Work out the finished part from the listing and answer in its coordinate system (mm). Coordinates: 2 decimals unless noted, no trailing zeros. Answer as a JSON object with one key per item and string values. Group by question number.
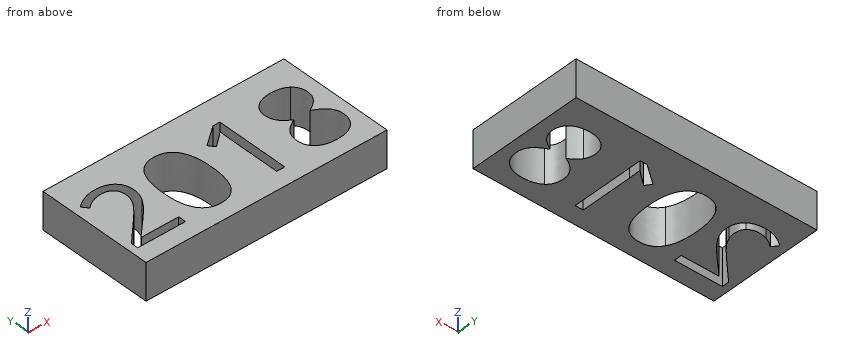
from build123d import *

# Parameters (mm, degrees)
F0_W     = 131.467973601
F0_H     = 63
F1_DEPTH = 20


with BuildPart() as f1:
    # F0 (on Top) → F1 (new body)
    with BuildSketch(Plane.XY):
        with Locations((-65.7339868005, -31.5)):
            Rectangle(F0_W, F0_H)
        with BuildLine():
            Line((-101.4531498872, -49.3273232344), (-101.4531498872, -53.5062699422))
            Line((-101.4531498872, -53.5062699422), (-127.5433306843, -53.5062699422))
            Line((-127.5433306843, -53.5062699422), (-127.5433306843, -49.6227165568))
            Line((-127.5433306843, -49.6227165568), (-117.0916198954, -39.1188775346))
            add(Edge.make_bspline(
                [(-117.0916198954, -39.1188775346), (-112.313198504, -34.279639871), (-110.7927916977, -32.2162306338)],
                knots=[0, 0, 0, 1, 1, 1], degree=2))
            add(Edge.make_bspline(
                [(-110.7927916977, -32.2162306338), (-109.2723848913, -30.1528213966), (-108.5121814882, -28.1980126456)],
                knots=[0, 0, 0, 1, 1, 1], degree=2))
            add(Edge.make_bspline(
                [(-108.5121814882, -28.1980126456), (-107.751978085, -26.2432038945), (-107.751978085, -23.9930018211)],
                knots=[0, 0, 0, 1, 1, 1], degree=2))
            add(Edge.make_bspline(
                [(-107.751978085, -23.9930018211), (-107.751978085, -20.8131795861), (-109.6807227193, -18.9539392629)],
                knots=[0, 0, 0, 1, 1, 1], degree=2))
            add(Edge.make_bspline(
                [(-109.6807227193, -18.9539392629), (-111.6094673537, -17.0946989397), (-115.0325546777, -17.0946989397)],
                knots=[0, 0, 0, 1, 1, 1], degree=2))
            add(Edge.make_bspline(
                [(-115.0325546777, -17.0946989397), (-117.4999577234, -17.0946989397), (-119.7154076413, -17.9113745957)],
                knots=[0, 0, 0, 1, 1, 1], degree=2))
            add(Edge.make_bspline(
                [(-119.7154076413, -17.9113745957), (-121.9308575591, -18.7280502517), (-124.6415256938, -20.8739958584)],
                knots=[0, 0, 0, 1, 1, 1], degree=2))
            Line((-124.6415256938, -20.8739958584), (-127.0307363895, -17.807118129))
            add(Edge.make_bspline(
                [(-127.0307363895, -17.807118129), (-121.5485838478, -13.2458977099), (-115.084682911, -13.2458977099)],
                knots=[0, 0, 0, 1, 1, 1], degree=2))
            add(Edge.make_bspline(
                [(-115.084682911, -13.2458977099), (-109.4895858637, -13.2458977099), (-106.3141076481, -16.1086065253)],
                knots=[0, 0, 0, 1, 1, 1], degree=2))
            add(Edge.make_bspline(
                [(-106.3141076481, -16.1086065253), (-103.1386294325, -18.9713153407), (-103.1386294325, -23.8018649655)],
                knots=[0, 0, 0, 1, 1, 1], degree=2))
            add(Edge.make_bspline(
                [(-103.1386294325, -23.8018649655), (-103.1386294325, -27.5811618841), (-105.2585109226, -31.2735784139)],
                knots=[0, 0, 0, 1, 1, 1], degree=2))
            add(Edge.make_bspline(
                [(-105.2585109226, -31.2735784139), (-107.3783924126, -34.9659949436), (-113.1820023934, -40.6132202243)],
                knots=[0, 0, 0, 1, 1, 1], degree=2))
            Line((-113.1820023934, -40.6132202243), (-121.8700412868, -49.1101222621))
            Line((-121.8700412868, -49.1101222621), (-121.8700412868, -49.3273232344))
            Line((-121.8700412868, -49.3273232344), (-101.4531498872, -49.3273232344))
        make_face(mode=Mode.SUBTRACT)
        with BuildLine():
            add(Edge.make_bspline(
                [(-72.7999976166, -18.4283129099), (-69.4464146037, -23.6715443821), (-69.4464146037, -33.6019728373)],
                knots=[0, 0, 0, 1, 1, 1], degree=2))
            add(Edge.make_bspline(
                [(-69.4464146037, -33.6019728373), (-69.4464146037, -43.897298926), (-72.6913971304, -48.9754576593)],
                knots=[0, 0, 0, 1, 1, 1], degree=2))
            add(Edge.make_bspline(
                [(-72.6913971304, -48.9754576593), (-75.9363796571, -54.0536163925), (-82.6174815662, -54.0536163925)],
                knots=[0, 0, 0, 1, 1, 1], degree=2))
            add(Edge.make_bspline(
                [(-82.6174815662, -54.0536163925), (-89.0205662307, -54.0536163925), (-92.3611171852, -48.8538251148)],
                knots=[0, 0, 0, 1, 1, 1], degree=2))
            add(Edge.make_bspline(
                [(-92.3611171852, -48.8538251148), (-95.7016681398, -43.654033837), (-95.7016681398, -33.6019728373)],
                knots=[0, 0, 0, 1, 1, 1], degree=2))
            add(Edge.make_bspline(
                [(-95.7016681398, -33.6019728373), (-95.7016681398, -23.2371424374), (-92.4697176714, -18.2111119375)],
                knots=[0, 0, 0, 1, 1, 1], degree=2))
            add(Edge.make_bspline(
                [(-92.4697176714, -18.2111119375), (-89.237767203, -13.1850814377), (-82.6174815662, -13.1850814377)],
                knots=[0, 0, 0, 1, 1, 1], degree=2))
            add(Edge.make_bspline(
                [(-82.6174815662, -13.1850814377), (-76.1535806295, -13.1850814377), (-72.7999976166, -18.4283129099)],
                knots=[0, 0, 0, 1, 1, 1], degree=2))
        make_face(mode=Mode.SUBTRACT)
        with BuildLine():
            Line((-47.2745393476, -13.810620238), (-47.2745393476, -53.5062699422))
            Line((-47.2745393476, -53.5062699422), (-51.6706870277, -53.5062699422))
            Line((-51.6706870277, -53.5062699422), (-51.6706870277, -25.2180153051))
            add(Edge.make_bspline(
                [(-51.6706870277, -25.2180153051), (-51.6706870277, -21.6819834755), (-51.4534860554, -18.536913396)],
                knots=[0, 0, 0, 1, 1, 1], degree=2))
            add(Edge.make_bspline(
                [(-51.4534860554, -18.536913396), (-52.0182085835, -19.110323963), (-52.7262837533, -19.7315187439)],
                knots=[0, 0, 0, 1, 1, 1], degree=2))
            add(Edge.make_bspline(
                [(-52.7262837533, -19.7315187439), (-53.4343589231, -20.3527135248), (-59.1858406706, -25.0268784495)],
                knots=[0, 0, 0, 1, 1, 1], degree=2))
            Line((-59.1858406706, -25.0268784495), (-61.5750513663, -21.9339366034))
            Line((-61.5750513663, -21.9339366034), (-51.0712123441, -13.810620238))
            Line((-51.0712123441, -13.810620238), (-47.2745393476, -13.810620238))
        make_face(mode=Mode.SUBTRACT)
        with BuildLine():
            add(Edge.make_bspline(
                [(-27.5787551762, -15.8088691835), (-24.3902449023, -13.2458977099), (-19.0384129439, -13.2458977099)],
                knots=[0, 0, 0, 1, 1, 1], degree=2))
            add(Edge.make_bspline(
                [(-19.0384129439, -13.2458977099), (-13.6083886355, -13.2458977099), (-10.43291042, -15.7697730085)],
                knots=[0, 0, 0, 1, 1, 1], degree=2))
            add(Edge.make_bspline(
                [(-10.43291042, -15.7697730085), (-7.2574322044, -18.293648307), (-7.2574322044, -22.7419242205)],
                knots=[0, 0, 0, 1, 1, 1], degree=2))
            add(Edge.make_bspline(
                [(-7.2574322044, -22.7419242205), (-7.2574322044, -25.6784813665), (-9.0732323331, -28.0937561788)],
                knots=[0, 0, 0, 1, 1, 1], degree=2))
            add(Edge.make_bspline(
                [(-9.0732323331, -28.0937561788), (-10.8890324619, -30.5090309912), (-14.8855303528, -32.4899038589)],
                knots=[0, 0, 0, 1, 1, 1], degree=2))
            add(Edge.make_bspline(
                [(-14.8855303528, -32.4899038589), (-10.0549807281, -34.8009222046), (-8.0176356076, -37.3378295615)],
                knots=[0, 0, 0, 1, 1, 1], degree=2))
            add(Edge.make_bspline(
                [(-8.0176356076, -37.3378295615), (-5.9802904871, -39.8747369184), (-5.9802904871, -43.2196318924)],
                knots=[0, 0, 0, 1, 1, 1], degree=2))
            add(Edge.make_bspline(
                [(-5.9802904871, -43.2196318924), (-5.9802904871, -48.1544379838), (-9.4294419278, -51.1040271882)],
                knots=[0, 0, 0, 1, 1, 1], degree=2))
            add(Edge.make_bspline(
                [(-9.4294419278, -51.1040271882), (-12.8785933685, -54.0536163925), (-18.8733402049, -54.0536163925)],
                knots=[0, 0, 0, 1, 1, 1], degree=2))
            add(Edge.make_bspline(
                [(-18.8733402049, -54.0536163925), (-25.2242966361, -54.0536163925), (-28.6473839601, -51.2690999271)],
                knots=[0, 0, 0, 1, 1, 1], degree=2))
            add(Edge.make_bspline(
                [(-28.6473839601, -51.2690999271), (-32.0704712841, -48.4845834618), (-32.0704712841, -43.3760165924)],
                knots=[0, 0, 0, 1, 1, 1], degree=2))
            add(Edge.make_bspline(
                [(-32.0704712841, -43.3760165924), (-32.0704712841, -36.5645941), (-23.764706102, -32.7592330646)],
                knots=[0, 0, 0, 1, 1, 1], degree=2))
            add(Edge.make_bspline(
                [(-23.764706102, -32.7592330646), (-27.509250865, -30.6480396135), (-29.1382581576, -28.1893246067)],
                knots=[0, 0, 0, 1, 1, 1], degree=2))
            add(Edge.make_bspline(
                [(-29.1382581576, -28.1893246067), (-30.7672654501, -25.7306095998), (-30.7672654501, -22.6897959871)],
                knots=[0, 0, 0, 1, 1, 1], degree=2))
            add(Edge.make_bspline(
                [(-30.7672654501, -22.6897959871), (-30.7672654501, -18.3718406571), (-27.5787551762, -15.8088691835)],
                knots=[0, 0, 0, 1, 1, 1], degree=2))
        make_face(mode=Mode.SUBTRACT)
    extrude(amount=-F1_DEPTH)


solid = f1.part
Q1. A flat-ended cylindrical pin translates along its axis: pin 1 Ø3 at (x, y) = (-49.5, -48) entering from +Z. Find the tip coordinate at first contact, or state that the pin passes through.
Q2. Consider L1, parallel to Y at x = -47.5, z = -0.75; L2, parallel to X at y = -43, z = -9; L3, parallel to Y at x = -124.5, z = -4.5. Determine where each line is inside the solid, lowest interval first. Write a range as from..to.
Q3. Section A-A on z = -7.25 is taken. Count the separate pieces of the cut face and the enclosed holes in it, plus the area to 3 significant figures.
Numbers:
{
 "1": {"pin 1": "passes through"},
 "2": {"L1": "y = -63..-53.51, -13.81..0", "L2": "x = -131.47..-120.95, -115.62..-94.74, -70.35..-51.67, -47.27..-32.06, -5.98..0", "L3": "y = -63..-53.51, -46.56..-20.76, -15.98..0"},
 "3": {"separate pieces": "1", "enclosed holes": "4", "area": "6,000 mm²"}
}
